Design review of the part built by this model. Coordinates are the model's own, in mm. Face numbers are marked on the shaded views. A direction names the side the tool comes from. Coordinates: 2 decimals unless noted, no trailing zeros. Write each loop counter-clockwise with the first axis right and the second up, starting at its lowest first coordinate (ties: lowest second). Pieces come first, ordered by that corner, then holes. Notation, with made-up numbers: (-17, -20.5) - (35, -20.5) arc R12 ccw to (35, -9.5) - close; hole circle Ø4 at (9.5, 9). An arc over 180 degrees is marked (long way). One line per item, written item: value.
from build123d import *

# Parameters (mm, degrees)
SKETCH1_W       = 7.96
SKETCH1_H       = 7.96
EXTRUDE1_DEPTH  = 9.7
SKETCH2_R       = 2.425
EXTRUDE2_DEPTH  = 1.8
LPATTERN1_COUNT = 2
LPATTERN1_PITCH = 7.96
SHELL1_T        = -1.55
SKETCH3_W       = 12.82
SKETCH3_H       = 4.86
EXTRUDE3_DEPTH  = 0.14
SKETCH4_R       = 1.5
EXTRUDE4_DEPTH  = 8.29
SKETCH5_W       = 1
SKETCH5_H       = 4.86
EXTRUDE5_DEPTH  = 6.29
EXTRUDE6_DEPTH  = 16.92
LPATTERN2_COUNT = 7
LPATTERN2_PITCH = 1.6
EXTRUDE7_DEPTH  = 10.7
LPATTERN3_COUNT = 11
LPATTERN3_PITCH = 1.6


with BuildPart() as part:
    # Sketch1 → Extrude1 (new body)
    with BuildSketch(Plane(origin=(0, 0, 0), x_dir=(1, 0, 0), z_dir=(0, 1, 0))):
        Rectangle(SKETCH1_W, SKETCH1_H)
    extrude1 = extrude(amount=EXTRUDE1_DEPTH)

    # Sketch2 → Extrude2 (add)
    with BuildSketch(Plane(origin=(0, 9.7, 0), x_dir=(1, 0, 0), z_dir=(0, 1, 0))):
        Circle(SKETCH2_R)
    extrude2 = extrude(amount=EXTRUDE2_DEPTH)

    # LPattern1: Extrude1, Extrude2 ×2
    with Locations(*[(i * LPATTERN1_PITCH, 0, 0) for i in range(1, LPATTERN1_COUNT)]):
        add(extrude1)
        add(extrude2)

    # Shell1
    shell1_openings = [part.faces().sort_by_distance(p)[0] for p in [
        (3.98, 0, 0),
    ]]
    offset(amount=SHELL1_T, openings=shell1_openings, kind=Kind.INTERSECTION)

    # Sketch3 → Extrude3 (cut)
    with BuildSketch(Plane.XZ.offset(-8.15)):
        with Locations((3.98, 0)):
            Rectangle(SKETCH3_W, SKETCH3_H)
    extrude(amount=-EXTRUDE3_DEPTH, mode=Mode.SUBTRACT)

    # Sketch4 → Extrude4 (add)
    with BuildSketch(Plane.XZ.offset(-8.29)):
        with Locations((3.98, 0)):
            Circle(SKETCH4_R)
    extrude(amount=EXTRUDE4_DEPTH)

    # Sketch5 → Extrude5 (add)
    with BuildSketch(Plane.XZ.offset(-8.29)):
        with Locations((3.98, 0)):
            Rectangle(SKETCH5_W, SKETCH5_H)
    extrude(amount=EXTRUDE5_DEPTH)

    # Sketch7 → Extrude6 (cut, through all)
    with BuildSketch(Plane(origin=(11.94, 0, 0), x_dir=(0, 0, -1), z_dir=(1, 0, 0))):
        Polygon((-3.98, -0.8), (-3.18, 0), (-3.98, 0.8), align=None)
    extrude6 = extrude(amount=-EXTRUDE6_DEPTH, mode=Mode.SUBTRACT)

    # LPattern2: Extrude6 ×7
    with Locations(*[(0, i * LPATTERN2_PITCH, 0) for i in range(1, LPATTERN2_COUNT)]):
        add(extrude6, mode=Mode.SUBTRACT)

    # Sketch8 → Extrude7 (cut, through all)
    with BuildSketch(Plane(origin=(0, 9.7, 0), x_dir=(1, 0, 0), z_dir=(0, 1, 0))):
        Polygon((-3.98, 3.18), (-3.18, 3.98), (-4.78, 3.98), align=None)
    extrude7 = extrude(amount=-EXTRUDE7_DEPTH, mode=Mode.SUBTRACT)

    # LPattern3: Extrude7 ×11
    with Locations(*[(i * LPATTERN3_PITCH, 0, 0) for i in range(1, LPATTERN3_COUNT)]):
        add(extrude7, mode=Mode.SUBTRACT)


solid = part.part
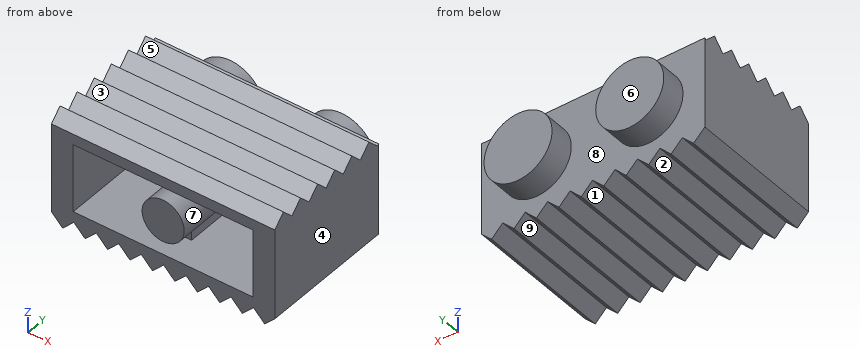
1. For the marked faces 5, 6, 7, 8 and 9, list the 3-axis set-ups (+Z, -Z, +X, -X, +Y, -Y) from which the entire face can be reached by the end or side of a thin tool; tool diameter is ignored.
Answer block:
face 5: +Z, +X, -X
face 6: +Z, -Z, +X, -X, +Y
face 7: -Y
face 8: +Y
face 9: -Z, +Y, -Y
2. Consider section D-D, the plane z = 0. Write out the cut boundary in (x, y) (3 decimals).
Answer block:
outline: (-3.98, 0) - (-2.43, 0) - (-2.43, 8.29) - (-0.875, 8.29) - (-0.875, 9.95) - (0.875, 9.95) - (0.875, 8.29) - (2.48, 8.29) - (2.48, 0) - (5.48, 0) - (5.48, 8.29) - (7.085, 8.29) - (7.085, 9.95) - (8.835, 9.95) - (8.835, 8.29) - (10.39, 8.29) - (10.39, 0) - (11.94, 0) - (11.94, 9.7) - (10.385, 9.7) - (10.385, 11.5) - (5.535, 11.5) - (5.535, 9.7) - (2.425, 9.7) - (2.425, 11.5) - (-2.425, 11.5) - (-2.425, 9.7) - (-3.98, 9.7) - close
3. Mouldability with a two-part tool opening along X and no side actions: class the marked faces 1, 2, 3 and 4 as released by +X, released by -X, zero draft, split by the parting line, or undercut.
Answer block:
face 1: undercut
face 2: undercut
face 3: zero draft
face 4: released by +X
4. Consider section A-A, the plane y = 1. Write out the cut boundary in (x, z), then the cut area to 3 significant figures.
Answer block:
outline: (-3.98, -3.18) - (-3.18, -3.98) - (-2.38, -3.18) - (-1.58, -3.98) - (-0.78, -3.18) - (0.02, -3.98) - (0.82, -3.18) - (1.62, -3.98) - (2.42, -3.18) - (3.22, -3.98) - (4.02, -3.18) - (4.82, -3.98) - (5.62, -3.18) - (6.42, -3.98) - (7.22, -3.18) - (8.02, -3.98) - (8.82, -3.18) - (9.62, -3.98) - (10.42, -3.18) - (11.22, -3.98) - (11.94, -3.26) - (11.94, 3.78) - (-3.98, 3.78) - close; circle Ø3 at (3.98, 0); hole (-2.43, -2.43) - (10.39, -2.43) - (10.39, 2.43) - (-2.43, 2.43) - close
area: 62.0 mm^2
5. Consider section C-C, the plane x = 6.75. Write out the cut boundary in (y, z).
Answer block:
outline: (0, -3.65) - (9.7, -3.65) - (9.7, -2.1) - (11.5, -2.1) - (11.5, 2.1) - (9.7, 2.1) - (9.7, 3.28) - (9.6, 3.18) - (8.8, 3.98) - (8, 3.18) - (7.2, 3.98) - (6.4, 3.18) - (5.6, 3.98) - (4.8, 3.18) - (4, 3.98) - (3.2, 3.18) - (2.4, 3.98) - (1.6, 3.18) - (0.8, 3.98) - (0, 3.18) - (0, 2.43) - (8.29, 2.43) - (8.29, -2.43) - (0, -2.43) - close
6. Insertion check: pin 1 Ø0.9 at (x, z) = (8.5, 0) entering from -Y; pin 2 Ø0.5 at (x, z) = (0, -0.5) entering from -Y; pin 3 Ø1 at (x, y) = (3.5, 3) entering from +Z. Each pin has a flat end and moves straight along its axis. Give the tip position at first contact, or say it passes through.
Answer block:
pin 1: stops at y = 8.29
pin 2: stops at y = 9.95
pin 3: stops at z = 3.88
7. Wall thickness on line 1 along X through (y, z) = (2.5, 0.5); line 2 along Y through (x, z) = (9.5, 3.5); line 3 along X through (y, z) = (6, -1): over which ranges is each line inside the solid? List them lowest first.
Answer block:
line 1: x = -3.98 to -2.43, 2.57 to 5.39, 10.39 to 11.94
line 2: y = 0.32 to 1.28, 1.92 to 2.88, 3.52 to 4.48, 5.12 to 6.08, 6.72 to 7.68, 8.32 to 9.28
line 3: x = -3.98 to -2.43, 2.86 to 5.1, 10.39 to 11.94
8. Consider section B-B, the plane z = -1.75. Write out the cut boundary in (x, y), then the cut area to 3 significant figures.
Answer block:
outline: (-3.98, 0) - (-2.43, 0) - (-2.43, 8.29) - (3.48, 8.29) - (3.48, 2) - (4.48, 2) - (4.48, 8.29) - (10.39, 8.29) - (10.39, 0) - (11.94, 0) - (11.94, 9.7) - (9.64, 9.7) - (9.64, 11.5) - (6.28, 11.5) - (6.28, 9.7) - (1.68, 9.7) - (1.68, 11.5) - (-1.68, 11.5) - (-1.68, 9.7) - (-3.98, 9.7) - close
area: 66.5 mm^2
